For this review, take the finished solid that the model builds, in its own axes (mm). A direction names the side the tool comes from. Round coordinates to 2 decimals unless told otherwise and drop trailing zeros. Order: outer loops, then holes, each group sorted by start corner. A loop starts at its lowest first (then second) coordinate and runs counter-clockwise, first axis right, second up. Notation, with made-up numbers: (-10.75, -16) - (9.25, -16) arc R23 cw to (9.25, 6) - close; hole circle Ø5 at (-39, 66). An arc over 180 degrees is marked (long way). Write each question's results on one line, items separated by ' | '. Start each with the question number.
(1) Take a section at A-A, the plane y = -45. Give the boundary of the cut face in (x, z).
(2) Insertion check: pin 1 Ø4 at (x, y) = (-9, -21) entering from +Z. The pin has a flat end and moves straight along its axis. Give the tip position at first contact, or say it passes through.
(3) Take a section at C-C, the plane x = -25. Give the boundary of the cut face in (y, z), plus the area to 3 significant figures.
(4) Take a section at D-D, the plane y = -21. Give the boundary of the cut face in (x, z).
(5) Take a section at B-B, the plane z = 3.75. Give the number of separate pieces and of enclosed holes in the cut face, plus the area to 3 significant figures.
(6) For L1, parallel to Y at x = 9, z = 2; L2, parallel to Y at x = -9, z = 7.2; L3, parallel to Y at x = 23, z = 7, list the stretches that pass through material, from the lowest coordinate up. Write a range as from..to.
(7) Draft analysis for pull direction X (two halves, no side actions). For faces 3 (the flat face through (9.7, 19.5, 6)), 4 (the flat face through (0, -50, 5)), 5 (the flat face through (-8.3, 43.5, 6)), state which applies: pulls with the +X half, pulls with the -X half, needs draft (parallel to the pull), parting line crosses it, or undercut.
(8) For faces 1 (the cylindrical face through (8.55, -17.58, 8.03)), 2 (the cylindrical face through (-7.89, 22.01, 2.96)), list the 3-axis set-ups (+Z, -Z, +X, -X, +Y, -Y) from which the entire face can be reached by the end or side of a thin tool; tool diameter is ignored.
```python
from build123d import *

# Parameters (mm, degrees)
SKETCH1_W           = 70
SKETCH1_H           = 100
BOSS_EXTRUDE1_DEPTH = 10
SKETCH2_R           = 2.5
CUT_EXTRUDE1_DEPTH  = 11
SKETCH3_R           = 1.5
CUT_EXTRUDE2_DEPTH  = 11
SKETCH4_R           = 3.45
CUT_EXTRUDE3_DEPTH  = 4


with BuildPart() as part:
    # Sketch1 → Boss-Extrude1 (new body)
    with BuildSketch(Plane.XY):
        Rectangle(SKETCH1_W, SKETCH1_H)
    extrude(amount=BOSS_EXTRUDE1_DEPTH)

    # Sketch2 → Cut-Extrude1 (cut, through all)
    with BuildSketch(Plane(origin=(0, 0, 0), x_dir=(-1, 0, 0), z_dir=(0, 0, -1))):
        with Locations((-25, 45)):
            Circle(SKETCH2_R)
        with Locations((25, 45)):
            Circle(SKETCH2_R)
        with Locations((-25, -45)):
            Circle(SKETCH2_R)
        with Locations((25, -45)):
            Circle(SKETCH2_R)
    extrude(amount=-CUT_EXTRUDE1_DEPTH, mode=Mode.SUBTRACT)

    # Sketch3 → Cut-Extrude2 (cut, through all)
    with BuildSketch(Plane(origin=(0, 0, 0), x_dir=(-1, 0, 0), z_dir=(0, 0, -1))):
        with Locations((9, 21)):
            Circle(SKETCH3_R)
        with Locations((9, 45)):
            Circle(SKETCH3_R)
        with Locations((-9, 21)):
            Circle(SKETCH3_R)
        with Locations((-9, 45)):
            Circle(SKETCH3_R)
        with Locations((9, -45)):
            Circle(SKETCH3_R)
        with Locations((9, -21)):
            Circle(SKETCH3_R)
        with Locations((-9, -45)):
            Circle(SKETCH3_R)
        with Locations((-9, -21)):
            Circle(SKETCH3_R)
    extrude(amount=-CUT_EXTRUDE2_DEPTH, mode=Mode.SUBTRACT)

    # Sketch4 → Cut-Extrude3 (cut)
    with BuildSketch(Plane.XY.offset(10)):
        with Locations((-9, 45)):
            Circle(SKETCH4_R)
        with Locations((-9, 21)):
            Circle(SKETCH4_R)
        with Locations((9, 21)):
            Circle(SKETCH4_R)
        with Locations((9, 45)):
            Circle(SKETCH4_R)
        with Locations((9, -21)):
            Circle(SKETCH4_R)
        with Locations((-9, -21)):
            Circle(SKETCH4_R)
        with Locations((-9, -45)):
            Circle(SKETCH4_R)
        with Locations((9, -45)):
            Circle(SKETCH4_R)
    extrude(amount=-CUT_EXTRUDE3_DEPTH, mode=Mode.SUBTRACT)


solid = part.part
```
Results below:
1) outline: (-35, 0) - (-27.5, 0) - (-27.5, 10) - (-35, 10) - close; (-22.5, 0) - (-10.5, 0) - (-10.5, 6) - (-12.45, 6) - (-12.45, 10) - (-22.5, 10) - close; (-7.5, 0) - (7.5, 0) - (7.5, 6) - (5.55, 6) - (5.55, 10) - (-5.55, 10) - (-5.55, 6) - (-7.5, 6) - close; (10.5, 0) - (22.5, 0) - (22.5, 10) - (12.45, 10) - (12.45, 6) - (10.5, 6) - close; (27.5, 0) - (35, 0) - (35, 10) - (27.5, 10) - close
2) pin 1: stops at z = 6
3) outline: (-50, 0) - (-47.5, 0) - (-47.5, 10) - (-50, 10) - close; (-42.5, 0) - (42.5, 0) - (42.5, 10) - (-42.5, 10) - close; (47.5, 0) - (50, 0) - (50, 10) - (47.5, 10) - close | area: 900 mm^2
4) outline: (-35, 0) - (-10.5, 0) - (-10.5, 6) - (-12.45, 6) - (-12.45, 10) - (-35, 10) - close; (-7.5, 0) - (7.5, 0) - (7.5, 6) - (5.55, 6) - (5.55, 10) - (-5.55, 10) - (-5.55, 6) - (-7.5, 6) - close; (10.5, 0) - (35, 0) - (35, 10) - (12.45, 10) - (12.45, 6) - (10.5, 6) - close
5) separate pieces: 1 | enclosed holes: 12 | area: 6,860 mm^2
6) L1: y = -50..-46.5, -43.5..-22.5, -19.5..19.5, 22.5..43.5, 46.5..50 | L2: y = -50..-48.45, -41.55..-24.45, -17.55..17.55, 24.45..41.55, 48.45..50 | L3: y = -50..-46.5, -43.5..43.5, 46.5..50
7) face 3: undercut | face 4: needs draft | face 5: undercut
8) face 1: +Z | face 2: +Z, -Z
